Check sheet for the modelled part. Datum: model origin and axes. Units: mm. Face numbers are marked on the shaded views. A direction names the side the tool comes from. Coordinates: 2 decimals unless noted, no trailing zeros. Write each loop counter-clockwise with the first axis right and the second up, starting at its lowest first coordinate (ties: lowest second). Pieces come first, ordered by that corner, then holes. Notation, with made-up numbers: (13, -23.75) -> (58, -23.75) arc R30 cw to (58, 11.25) -> close; hole circle Ø8 at (-39.5, -7.5). An arc over 180 degrees is marked (long way). Put each result on its own line as item: value.
```python
from build123d import *

# Parameters (mm, degrees)
F0_W      = 25
F0_H      = 6.5
F0_R      = 1.85
F1_DEPTH  = 5
F3_DEPTH  = 2.1
F5_DEPTH  = 8.2
F7_DEPTH  = 5
F9_DEPTH  = 2
F11_DEPTH = 2
F12_R     = 1.85
F13_DEPTH = 5
F14_R     = 1.85
F15_DEPTH = 5
F17_DEPTH = 2


# Not quite as in the source:
# - a feature names something its author has since deleted; it is built from what else it names


with BuildPart() as f1:
    # F0 (on Top) → F1 (new body)
    with BuildSketch(Plane.XY):
        with BuildLine():
            Line((-14.9, 24), (-20, 24))
            Line((-20, 24), (-20, -11))
            Line((-20, -11), (-12.5, -11))
            Line((-12.5, -11), (12.5, -11))
            Line((12.5, -11), (20, -11))
            Line((20, -11), (20, 24))
            Line((20, 24), (14.9, 24))
            Line((14.9, 24), (14.9, 9.4))
            ThreePointArc((14.9, 9.4), (0, -5.5), (-14.9, 9.4))
            Line((-14.9, 9.4), (-14.9, 24))
        make_face()
        with Locations((0, -14.25)):
            Rectangle(F0_W, F0_H)
        with Locations((0, -12.9)):
            Circle(F0_R, mode=Mode.SUBTRACT)
    extrude(amount=F1_DEPTH)

    # F2 (on face) → F3 (join)
    with BuildSketch(Plane.XY.offset(5)):
        with BuildLine():
            Line((-14.9, 24), (-20, 24))
            Line((-20, 24), (-20, -11))
            Line((-20, -11), (20, -11))
            Line((20, -11), (20, 24))
            Line((20, 24), (14.9, 24))
            Line((14.9, 24), (14.9, 9.4))
            ThreePointArc((14.9, 9.4), (0, -5.5), (-14.9, 9.4))
            Line((-14.9, 9.4), (-14.9, 24))
        make_face()
    extrude(amount=F3_DEPTH)

    # F4 (on face) → F5 (join)
    with BuildSketch(Plane.XY.offset(7.1)):
        with BuildLine():
            Line((-17.35, 24), (-20, 24))
            Line((-20, 24), (-20, -11))
            Line((-20, -11), (20, -11))
            Line((20, -11), (20, 24))
            Line((20, 24), (17.35, 24))
            Line((17.35, 24), (17.35, 9.4))
            ThreePointArc((17.35, 9.4), (0, -7.95), (-17.35, 9.4))
            Line((-17.35, 9.4), (-17.35, 24))
        make_face()
    extrude(amount=F5_DEPTH)

    # F6 (on face) → F7 (join)
    with BuildSketch(Plane.XY.offset(15.3)):
        with BuildLine():
            Line((-14.9, 24), (-20, 24))
            Line((-20, 24), (-20, -11))
            Line((-20, -11), (-15, -11))
            Line((-15, -11), (-15, -21))
            Line((-15, -21), (15, -21))
            Line((15, -21), (15, -11))
            Line((15, -11), (20, -11))
            Line((20, -11), (20, 24))
            Line((20, 24), (14.9, 24))
            Line((14.9, 24), (14.9, 9.4))
            ThreePointArc((14.9, 9.4), (0, -5.5), (-14.9, 9.4))
            Line((-14.9, 9.4), (-14.9, 24))
        make_face()
    extrude(amount=F7_DEPTH)

    # F8 (on face) → F9 (cut)
    with BuildSketch(Plane(origin=(-20, 0, 0), x_dir=(0, -1, 0), z_dir=(-1, 0, 0))):
        with BuildLine():
            ThreePointArc((-6.8885265259, 5.9499996589), (-6.5988151547, 6.649424579), (-6.5, 7.4))
            ThreePointArc((-6.5, 7.4), (-6.598815139, 8.1505753623), (-6.8885264651, 8.8500002357))
            ThreePointArc((-6.8885264651, 8.8500002357), (-7.9500001179, 9.911473739), (-9.4, 10.3))
            ThreePointArc((-9.4, 10.3), (-10.849999907, 9.9114737247), (-11.9114735636, 8.850000186))
            ThreePointArc((-11.9114735636, 8.850000186), (-12.3, 7.3999999856), (-11.9114735492, 5.9499997892))
            ThreePointArc((-11.9114735492, 5.9499997892), (-10.8499998946, 4.8885262682), (-9.4, 4.5))
            ThreePointArc((-9.4, 4.5), (-7.9500001705, 4.8885262306), (-6.8885265259, 5.9499996589))
        make_face()
        with BuildLine():
            ThreePointArc((-6.8885264651, 8.8500002357), (-6.598815139, 8.1505753623), (-6.5, 7.4))
            ThreePointArc((-6.5, 7.4), (-6.5988151547, 6.649424579), (-6.8885265259, 5.9499996589))
            Line((-6.8885265259, 5.9499996589), (-6.0513684387, 7.4))
            Line((-6.0513684387, 7.4), (-6.8885264651, 8.8500002357))
        make_face()
        with BuildLine():
            ThreePointArc((-9.4, 10.3), (-7.9500001179, 9.911473739), (-6.8885264651, 8.8500002357))
            Line((-6.8885264651, 8.8500002357), (-7.7256842194, 10.3))
            Line((-7.7256842194, 10.3), (-9.4, 10.3))
        make_face()
        with BuildLine():
            Line((-7.7256842194, 4.5), (-6.8885265259, 5.9499996589))
            ThreePointArc((-6.8885265259, 5.9499996589), (-7.9500001705, 4.8885262306), (-9.4, 4.5))
            Line((-9.4, 4.5), (-7.7256842194, 4.5))
        make_face()
        with BuildLine():
            ThreePointArc((-11.9114735636, 8.850000186), (-10.849999907, 9.9114737247), (-9.4, 10.3))
            Line((-9.4, 10.3), (-11.0743157806, 10.3))
            Line((-11.0743157806, 10.3), (-11.9114735636, 8.850000186))
        make_face()
        with BuildLine():
            Line((-11.0743157806, 4.5), (-9.4, 4.5))
            ThreePointArc((-9.4, 4.5), (-10.8499998946, 4.8885262682), (-11.9114735492, 5.9499997892))
            Line((-11.9114735492, 5.9499997892), (-11.0743157806, 4.5))
        make_face()
        with BuildLine():
            ThreePointArc((-11.9114735492, 5.9499997892), (-12.3, 7.3999999856), (-11.9114735636, 8.850000186))
            Line((-11.9114735636, 8.850000186), (-12.7486315613, 7.4))
            Line((-12.7486315613, 7.4), (-11.9114735492, 5.9499997892))
        make_face()
    extrude(amount=-F9_DEPTH, mode=Mode.SUBTRACT)

    # F10 (on face) → F11 (cut)
    with BuildSketch(Plane.YZ.offset(20)):
        Polygon((11.0743157806, 10.3), (7.7256842194, 10.3), (6.0513684387, 7.4), (7.7256842194, 4.5), (11.0743157806, 4.5), (12.7486315613, 7.4), align=None)
    extrude(amount=-F11_DEPTH, mode=Mode.SUBTRACT)

    # F12 (on face) → F13 (cut)
    with BuildSketch(Plane.YZ.offset(18)):
        with Locations((9.4, 7.4)):
            Circle(F12_R)
    extrude(amount=-F13_DEPTH, mode=Mode.SUBTRACT)

    # F14 (on face) → F15 (cut)
    with BuildSketch(Plane(origin=(-18, 0, 0), x_dir=(0, -1, 0), z_dir=(-1, 0, 0))):
        with Locations((-9.4, 7.4)):
            Circle(F14_R)
    extrude(amount=-F15_DEPTH, mode=Mode.SUBTRACT)

    # F16 (on Top) → F17 (cut)
    with BuildSketch(Plane.XY):
        Polygon((-1.6743157806, -15.8), (1.6743157806, -15.8), (3.3486315613, -12.9), (1.6743157806, -10), (-1.6743157806, -10), (-3.3486315613, -12.9), align=None)
    extrude(amount=F17_DEPTH, mode=Mode.SUBTRACT)


solid = f1.part
```
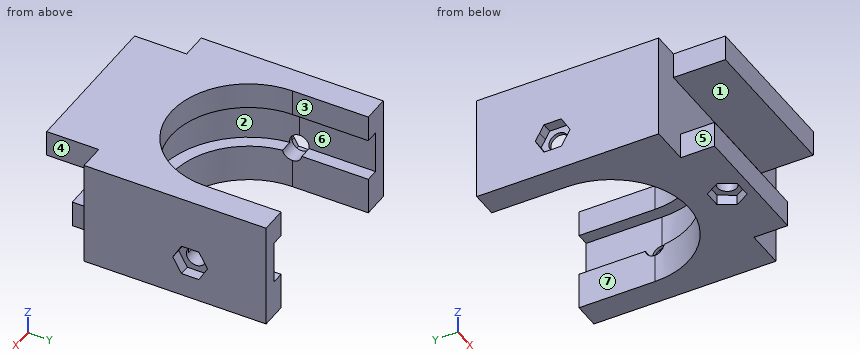
Q1. Material ranges on line 1 along Z through (x, y) = (16.5, 9.4); line 2 along X through (y, z) = (-12.9, 3.85); line 3 along X through (y, z) = (19, 8), recorded low to high.
Recorded:
line 1: z = 0 to 5.55, 15.3 to 20.3
line 2: x = -12.5 to -1.85, 1.85 to 12.5
line 3: x = -20 to -17.35, 17.35 to 20
Q2. Cross-section at B-B (x = 0). Record the cut outline in (y, z).
Recorded:
outline: (-21, 15.3) -> (-11, 15.3) -> (-11, 5) -> (-11.05, 5) -> (-11.05, 2) -> (-10, 2) -> (-10, 0) -> (-5.5, 0) -> (-5.5, 7.1) -> (-7.95, 7.1) -> (-7.95, 15.3) -> (-5.5, 15.3) -> (-5.5, 20.3) -> (-21, 20.3) -> close; (-17.5, 0) -> (-15.8, 0) -> (-15.8, 2) -> (-14.75, 2) -> (-14.75, 5) -> (-17.5, 5) -> close
Q3. Cross-section at D-D (z = 12.5). Record the cut outline in (x, y).
Recorded:
outline: (-20, -11) -> (20, -11) -> (20, 24) -> (17.35, 24) -> (17.35, 9.4) arc R17.35 cw to (-17.35, 9.4) -> (-17.35, 24) -> (-20, 24) -> close
Q4. Depth check by flat-ended pin: P1, Ø4, axis at y = -15, z = 3, coming from the -X side; P2, Ø6, axis at x = -1.5, z = 7, coming from the -Y side; P3, Ø1, axis at x = -7, z = 12, coming from the +Y side; P4, Ø12, axis at y = -15.5, z = 12.5, coming from the +X side. Enter the tip coordinate at first touch or a pass-through.
Recorded:
P1: stops at x = -12.5
P2: stops at y = -17.5
P3: stops at y = -6.25
P4: stops at x = 20
Q5. Cross-section at C-C (y = 19). Record the cut outline in (x, z).
Recorded:
outline: (-20, 0) -> (-14.9, 0) -> (-14.9, 7.1) -> (-17.35, 7.1) -> (-17.35, 15.3) -> (-14.9, 15.3) -> (-14.9, 20.3) -> (-20, 20.3) -> close; (14.9, 0) -> (20, 0) -> (20, 20.3) -> (14.9, 20.3) -> (14.9, 15.3) -> (17.35, 15.3) -> (17.35, 7.1) -> (14.9, 7.1) -> close
Q6. Tool access check on the marked faces 5, 6 and 7. Record the directions out of +Z, -Z, +X, -X, +Y, -Y that give a thin tool (end or side, any length) a straight path to the whole face; none if there is none.
Recorded:
face 5: -Z, -X, -Y
face 6: +Y
face 7: +Z, -Z, +Y
Q7. Cross-section at A-A (z = 3.25). Record the cut outline in (x, y).
Recorded:
outline: (-20, -11) -> (-12.5, -11) -> (-12.5, -17.5) -> (12.5, -17.5) -> (12.5, -11) -> (20, -11) -> (20, 24) -> (14.9, 24) -> (14.9, 9.4) arc R14.9 cw to (-14.9, 9.4) -> (-14.9, 24) -> (-20, 24) -> close; hole circle Ø3.7 at (0, -12.9)
Q8. Mould release check, pull along X, two halves, no side actions. Record for the marked faces 1, 2, 3 and 4: released by +X, released by -X, zero draft, split by the parting line, or undercut.
Recorded:
face 1: zero draft
face 2: undercut
face 3: undercut
face 4: released by +X
